Model file for the job. Use its own axes, mm. A direction names the side the tool comes from. Coordinates: 2 decimals unless noted, no trailing zeros. Loops run counter-clockwise (first coordinate to the right, second up) from the corner with the lowest first, then second, coordinate; pieces in that order, holes last.
from build123d import *

# Parameters (mm, degrees)
F1_DEPTH  = 16
F2_W      = 70
F2_H      = 3
F3_DEPTH  = 2
F4_W      = 50
F4_H      = 2
F4_H_2    = 12
F5_DEPTH  = 1
F6_R      = 1
F9_DEPTH  = 2
F11_DEPTH = 38.001
F13_D     = 4
F13_DEPTH = 50
F13_TIP   = 1.2017212381
F14_R     = 3
F14_R_2   = 2
F15_DEPTH = 5
F16_R     = 3


# Not quite as in the source:
# - a pattern or mirror of a feature is missing from the dataset's text; its kind, count and spacing are read off the source's solid


with BuildPart() as f1:
    # F0 (on Top) → F1 (new body)
    with BuildSketch(Plane.XY):
        with BuildLine():
            Line((94, 38.2990682213), (94, 40.2990682213))
            Line((94, 40.2990682213), (0, 40.2990682213))
            ThreePointArc((0, 40.2990682213), (-5.6829599791, 31.9326325705), (0, 23.5661969196))
            Line((0, 23.5661969196), (19, 23.5661969196))
            ThreePointArc((19, 23.5661969196), (22.2913263859, 22.330127129), (23.9553291252, 19.2330651681))
            ThreePointArc((23.9553291252, 19.2330651681), (55.0865893222, -19.5660123964), (104.1299821488, -27.8888365183))
            Line((104.1299821488, -27.8888365183), (104.1769053316, -27.8687567031))
            ThreePointArc((104.1769053316, -27.8687567031), (111.1768871923, -29.1372905243), (117.1067956471, -33.0673172193))
            Line((117.1067956471, -33.0673172193), (118.5684373125, -31.7009317787))
            ThreePointArc((118.5684373125, -31.7009317787), (109.440201014, -26.4706046683), (98.9222178887, -26.7009317787))
            ThreePointArc((98.9222178887, -26.7009317787), (60.1395132052, -20.0357341509), (31.5428701215, 6.9967471693))
            ThreePointArc((31.5428701215, 6.9967471693), (28.6246292953, 13.1964823258), (25.9374607753, 19.4998124675))
            ThreePointArc((25.9374607753, 19.4998124675), (23.6078569403, 23.8356992128), (19, 25.5661969196))
            Line((19, 25.5661969196), (0.4069717908, 25.5661969196))
            ThreePointArc((0.4069717908, 25.5661969196), (-3.6829599791, 31.9326325705), (0.4069717908, 38.2990682213))
            Line((0.4069717908, 38.2990682213), (94, 38.2990682213))
        make_face()
    extrude(amount=F1_DEPTH)

    # F2 (on face) → F3 (join)
    with BuildSketch(Plane(origin=(0, 40.2990682213, 0), x_dir=(-1, 0, 0), z_dir=(0, 1, 0))):
        with Locations((-59, 17.5)):
            Rectangle(F2_W, F2_H)
    extrude(amount=-F3_DEPTH)

    # F4 (on face) → F5 (join)
    with BuildSketch(Plane.XY.offset(19)):
        with Locations((69, 39.2990682213)):
            Rectangle(F4_W, F4_H)
        with Locations((69, 32.2990682213)):
            Rectangle(F4_W, F4_H_2)
    extrude(amount=-F5_DEPTH)

    # F6
    f6_edges = [f1.edges().sort_by_distance(p)[0] for p in [
        (59, 40.299068, 19),
    ]]
    fillet(f6_edges, radius=F6_R)

    # F7: F1 across face


with BuildPart() as f1_1:
    add(f1.part)
    add(f1.part.mirror(Plane(origin=(48.2414959272, 12.2129217621, 0), x_dir=(1, 0, 0), z_dir=(0, 0, -1))))

    # F8 (on face) → F9 (cut)
    with BuildSketch(Plane(origin=(0, 40.2990682213, 0), x_dir=(-1, 0, 0), z_dir=(0, 1, 0))):
        with BuildLine():
            Line((-34, 11.8147813603), (-94, 11.8147813603))
            Line((-94, 11.8147813603), (-94, -12.1852186397))
            Line((-94, -12.1852186397), (-34, -12.1852186397))
            ThreePointArc((-34, -12.1852186397), (-22, -0.1852186397), (-34, 11.8147813603))
        make_face()
    extrude(amount=-F9_DEPTH, mode=Mode.SUBTRACT)

    # F10 (on face) → F11 (cut, through all)
    with BuildSketch(Plane.XY.offset(19)):
        with BuildLine():
            ThreePointArc((50, 34.2990682213), (47, 31.2990682213), (50, 28.2990682213))
            Line((50, 28.2990682213), (70, 28.2990682213))
            ThreePointArc((70, 28.2990682213), (73, 31.2990682213), (70, 34.2990682213))
            Line((70, 34.2990682213), (50, 34.2990682213))
        make_face()
    extrude(amount=-F11_DEPTH, mode=Mode.SUBTRACT)

    # F13
    with Locations(Plane.XY.offset(19)):
        with Locations((80, 32.2990682213)):
            Hole(F13_D / 2, depth=F13_DEPTH)
            with Locations((0, 0, -(F13_DEPTH + F13_TIP / 2))):  # 118° drill point
                Cone(0, F13_D / 2, F13_TIP, mode=Mode.SUBTRACT)

    # F14 (on face) → F15 (join)
    with BuildSketch(Plane.XY.offset(19)):
        with Locations((80, 32.2990682213)):
            Circle(F14_R)
        with Locations((80, 32.2990682213)):
            Circle(F14_R_2, mode=Mode.SUBTRACT)
    f15 = extrude(amount=-F15_DEPTH)

    # F15_copies: F15 across plane
    add(f15.mirror(Plane(origin=(0, 0, 0), x_dir=(-1, 0, 0), z_dir=(0, 0, -1))))

    # F16
    f16_edges = [f1_1.edges().sort_by_distance(p)[0] for p in [
        (44, 26.299068, 18.5),
        (44, 26.299068, -18.5),
        (94, 26.299068, -18.5),
        (94, 26.299068, 18.5),
    ]]
    fillet(f16_edges, radius=F16_R)


solid = f1_1.part
Q1. Flat gauge pins, fed straight in: P1, Ø5, axis at x = 80, y = 32.3, coming from the -Z side; P2, Ø1.1, axis at x = 56.5, z = 18.5, coming from the -Y side; P3, Ø2, axis at y = 34.5, z = -15, coming from the +X side; P4, Ø12, axis at y = 8.5, z = -3, coming from the -X side. Where does each tip first touch, or does it go through?
Answers:
P1: stops at z = -19
P2: stops at y = 26.3
P3: stops at x = 82.75
P4: stops at x = 25.68
Q2. Drill centre lines: line 1 (Y direction, x = 80, z = 16.4); line 2 (Y direction, x = 4, z = 6.5); line 3 (Y direction, x = 80, z = 15.9). Where is each one in solid material? Low to high.
Answers:
line 1: y = 29.3 to 30.3, 34.3 to 35.3, 38.3 to 40.3
line 2: y = 23.57 to 25.57, 38.3 to 40.3
line 3: y = -28.42 to -26.39, 29.3 to 30.3, 34.3 to 35.3, 38.3 to 40.3
Q3. Slice it at C-C (z = 0). List the corners of the cut face in (x, y), and give its area (3 significant figures).
Answers:
outline: (0, 23.57) - (19, 23.57) arc R5 cw to (23.96, 19.23) arc R70 ccw to (104.13, -27.89) - (104.18, -27.87) arc R17.64 cw to (117.11, -33.07) - (118.57, -31.7) arc R19.64 ccw to (98.92, -26.7) arc R68 cw to (31.54, 7) arc R185.41 cw to (25.94, 19.5) arc R7 ccw to (19, 25.57) - (0.41, 25.57) arc R7 cw to (0.41, 38.3) - (22, 38.3) - (22, 40.3) - (0, 40.3) arc R9 ccw to start
area: 369 mm2
Q4. Slice it at A-A (x = 59). List the corners of the cut face in (y, z).
Answers:
outline: (-21.7, -16) - (-19.45, -16) - (-19.45, 16) - (-21.7, 16) - close; (26.3, -19) - (28.3, -19) - (28.3, -18) - (26.3, -18) - close; (26.3, 18) - (28.3, 18) - (28.3, 19) - (26.3, 19) - close; (34.3, -19) - (39.3, -19) arc R1 ccw to (40.3, -18) - (40.3, -12.19) - (38.3, -12.19) - (38.3, -18) - (34.3, -18) - close; (34.3, 18) - (38.3, 18) - (38.3, 11.81) - (40.3, 11.81) - (40.3, 18) arc R1 ccw to (39.3, 19) - (34.3, 19) - close
Q5. Slice it at B-B (x = 8). List the corners of the cut face in (y, z).
Answers:
outline: (23.57, -16) - (25.57, -16) - (25.57, 16) - (23.57, 16) - close; (38.3, -16) - (40.3, -16) - (40.3, 16) - (38.3, 16) - close
Q6. Slice it at D-D (x = 80). Count the separate pieces of the cut face and the enclosed holes in it, and give its area (3 significant figures).
Answers:
separate pieces: 5
enclosed holes: 0
area: 124 mm2
Q7. Mould opens along X. For faces 6 (the cylindrical face through (22.253, 22.363, 0.224)), 7 (the flat face through (9, 23.566, 0)), 8 (the cylindrical face through (73, 31.2, -18.5)) say: +X half, -X half, draft (parallel to the pull), parting line (faces both ways), or undercut.
Answers:
face 6: -X half
face 7: draft
face 8: undercut
Q8. Which spindle directions (+Z, -Z, +X, -X, +Y, -Y) get a long thin tool onto all of the face, cutting with end or side? Do faces 1 (the cylindrical face through (22, 39, 0)), 2 (the cylindrical face through (23.66, 23.79, 0.22)), 3 (the cylindrical face through (77.6, 30.5, 16)), 4 (the flat face through (81, 30, -14)), 5 (the cylindrical face through (60.64, -20.284, 0.224)). Say none if no direction does.
Answers:
face 1: +X, +Y
face 2: +Z, -Z, +X
face 3: none
face 4: +X
face 5: +Z, -Z
